Verification items for the finished model (mm, model axes). Coordinates: 2 decimals unless noted, no trailing zeros. Order: outer loops, then holes, each group sorted by start corner. A loop starts at its lowest first (then second) coordinate and runs counter-clockwise, first axis right, second up. Notation, with made-up numbers: (80.25, -7) - (109.25, -7) arc R7 ccw to (109.25, 6) - close; hole circle Ø10 at (-14, 84.25). An arc over 180 degrees is marked (long way). Answer as CSV lines item,"result". Start each with the question number.
1. Section check A-A (x = 90). Record the cut outline in (y, z).
2. Section check C-C (z = 2.4). Count the separate pieces of the cut face and the enclosed holes in it, and give its area (3 significant figures).
3. Section check D-D (x = -26). Record the cut outline in (y, z), and give its area (3 significant figures).
4. Material ranges on L1, parallel to X at y = 8, z = 0.95; L2, parallel to X at y = 14, z = 3.35; L3, parallel to X at y = 23, z = 3.5, recorded low to high. Write a range as [from, to].
5. Go/stop test with a flat-tipped pin: pin 1 (1.8 mm diameter, centred on x = -2, z = 3, fed in from -Y). Record where the tip stops, or that it passes through.
6. Section check B-B (x = 43). Record the cut outline in (y, z), and give its area (3 significant figures).
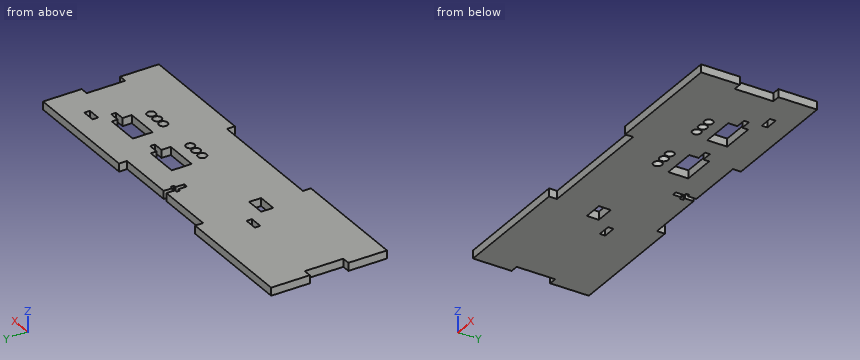
from build123d import *

# Parameters (mm, degrees)
SKETCH1_W           = 231.14
SKETCH1_H           = 73.66
BOSS_EXTRUDE1_DEPTH = 5.08
SKETCH2_W           = 77.046666666
SKETCH2_H           = 5.08
CUT_EXTRUDE1_DEPTH  = 122.402966191
SKETCH3_W           = 5.08
SKETCH3_H           = 24.553333334
CUT_EXTRUDE2_DEPTH  = 122.402966191
SKETCH5_W           = 2.7559
SKETCH5_H           = 13.081
CUT_EXTRUDE4_DEPTH  = 122.402966191
SKETCH6_W           = 6.096
SKETCH6_H           = 2.1717
CUT_EXTRUDE5_DEPTH  = 122.402966191
CAVITY1_OUTLINE_R   = 2.7305
CAVITY1_OUTLINE_W   = 12.202797109
CAVITY1_OUTLINE_H   = 7.62
CAVITY1_OUTLINE_W_2 = 8.382
CAVITY1_OUTLINE_H_2 = 3.429
CAVITY1_OUTLINE_H_3 = 3.556
CAVITY1_DEPTH       = 5.08


# Read off the part's stored shape, not the designer's step: Cavity1
with BuildPart() as part:
    # Sketch1 → Boss-Extrude1 (new body)
    with BuildSketch(Plane.XY):
        Rectangle(SKETCH1_W, SKETCH1_H)
    extrude(amount=BOSS_EXTRUDE1_DEPTH)

    # Sketch2 → Cut-Extrude1 (cut, through all)
    with BuildSketch(Plane.XY.offset(5.08)):
        with Locations((0, -34.29)):
            Rectangle(SKETCH2_W, SKETCH2_H)
        with Locations((0, 34.29)):
            Rectangle(SKETCH2_W, SKETCH2_H)
    extrude(amount=-CUT_EXTRUDE1_DEPTH, mode=Mode.SUBTRACT)

    # Sketch3 → Cut-Extrude2 (cut, through all)
    with BuildSketch(Plane.XY.offset(5.08)):
        with Locations((-113.03, 0)):
            Rectangle(SKETCH3_W, SKETCH3_H)
        with Locations((113.03, 0)):
            Rectangle(SKETCH3_W, SKETCH3_H)
    extrude(amount=-CUT_EXTRUDE2_DEPTH, mode=Mode.SUBTRACT)

    # Sketch5 → Cut-Extrude4 (cut, through all)
    with BuildSketch(Plane.XY.offset(5.08)):
        with Locations((0, 25.2095)):
            Rectangle(SKETCH5_W, SKETCH5_H)
    extrude(amount=-CUT_EXTRUDE4_DEPTH, mode=Mode.SUBTRACT)

    # Sketch6 → Cut-Extrude5 (cut, through all)
    with BuildSketch(Plane.XY.offset(5.08)):
        with Locations((0, 25.2095)):
            Rectangle(SKETCH6_W, SKETCH6_H)
    extrude(amount=-CUT_EXTRUDE5_DEPTH, mode=Mode.SUBTRACT)

    # Cavity1 outline → Cavity1 (cut)
    with BuildSketch(Plane.XY):
        with Locations((21.814879295, -5.588)):
            Circle(CAVITY1_OUTLINE_R)
        with Locations((27.972778565, -5.588)):
            Circle(CAVITY1_OUTLINE_R)
        with Locations((33.971893142, -5.588)):
            Circle(CAVITY1_OUTLINE_R)
        Polygon((38.577278565, 12.877703873), (38.577278565, 16.614191805), (17.368278565, 16.614191805), (17.368278565, 3.914191805), (38.577278565, 3.914191805), (38.577278565, 9.829703873), (45.181278565, 9.829703873), (45.181278565, 12.877703873), align=None)
        Polygon((56.847527144, 3.914191805), (78.056527144, 3.914191805), (78.056527144, 9.829703873), (84.660527144, 9.829703873), (84.660527144, 12.877703873), (78.056527144, 12.877703873), (78.056527144, 16.614191805), (56.847527144, 16.614191805), align=None)
        with Locations((61.294127875, -5.588)):
            Circle(CAVITY1_OUTLINE_R)
        with Locations((67.452027144, -5.588)):
            Circle(CAVITY1_OUTLINE_R)
        with Locations((73.451141721, -5.588)):
            Circle(CAVITY1_OUTLINE_R)
        with Locations((-38.971851196, -4.900880915)):
            Rectangle(CAVITY1_OUTLINE_W, CAVITY1_OUTLINE_H)
        with Locations((-53.192397728, 8.983802784)):
            Rectangle(CAVITY1_OUTLINE_W_2, CAVITY1_OUTLINE_H_2)
        with Locations((89.651170694, 22.423911141)):
            Rectangle(CAVITY1_OUTLINE_W_2, CAVITY1_OUTLINE_H_3)
    extrude(amount=CAVITY1_DEPTH, mode=Mode.SUBTRACT)


solid = part.part
Evaluation:
1,outline,"(-36.83, 0) - (20.65, 0) - (20.65, 5.08) - (-36.83, 5.08) - close; (24.2, 0) - (36.83, 0) - (36.83, 5.08) - (24.2, 5.08) - close"
2,separate pieces,"1"
2,enclosed holes,"11"
2,area,"15,100 mm²"
3,outline,"(-31.75, 0) - (31.75, 0) - (31.75, 5.08) - (-31.75, 5.08) - close"
3,area,"323 mm²"
4,L1,"x = [-110.49, -57.38], [-49, 17.37], [38.58, 56.85], [78.06, 110.49]"
4,L2,"x = [-115.57, 17.37], [38.58, 56.85], [78.06, 115.57]"
4,L3,"x = [-115.57, -1.38], [1.38, 85.46], [93.84, 115.57]"
5,pin 1,"stops at y = -31.75"
6,outline,"(-36.83, 0) - (9.83, 0) - (9.83, 5.08) - (-36.83, 5.08) - close; (12.88, 0) - (36.83, 0) - (36.83, 5.08) - (12.88, 5.08) - close"
6,area,"359 mm²"
